Build history of the part. All positions in model axes, mm. Face numbers are marked on the shaded views. A direction names the side the tool comes from. Give positions to 0.01 mm unless a question says otherwise; leave off trailing zeros. Order: outer loops, then holes, each group sorted by start corner. A loop starts at its lowest first (then second) coordinate and runs counter-clockwise, first axis right, second up. Notation, with made-up numbers: (2.5, 76.5) - (47.5, 76.5) arc R10 ccw to (47.5, 83.5) - close; hole circle Ø2 at (13, 10.25). An arc over 180 degrees is marked (long way). Write each question's results on one line, items separated by ' | '. Start each with the question number.
1) Drill centre lines: line 1 along Z through (x, y) = (19.5, 6); line 2 along Y through (x, z) = (0, 5); line 3 along X through (y, z) = (8.5, 3.5). Where is each one in solid material? Low to high. Write a range as from..to.
2) Tool access for the marked faces 1 and 2: list every direction of +Z, -Z, +X, -X, +Y, -Y with a clear straight run to the whole face (end or side of a thin tool).
3) Cut at A-A on x = 0. List the corners of the cut face in (y, z).
4) Cut at C-C on z = 23.5. List the corners of the cut face in (x, y), plus the area to 3 significant figures.
5) Drop flat-ended pins along their axis: pin 1 Ø6 at (x, z) = (9, 18.5) entering from -Y; pin 2 Ø5 at (y, z) = (-13.5, 11.5) entering from -X; pin 3 Ø4 at (y, z) = (-2.5, 6) entering from -X. Give the stop position or say it passes through.
from build123d import *

# Parameters (mm, degrees)
F0_R     = 24.25
F1_DEPTH = 25
F2_R     = 14.75
F3_DEPTH = 4.5
F4_SIZE  = 1


with BuildPart() as f1:
    # F0 (on Top) → F1 (new body)
    with BuildSketch(Plane.XY):
        Circle(F0_R)
    extrude(amount=F1_DEPTH)

    # F2 (on face) → F3 (join)
    with BuildSketch(Plane.XY.offset(25)):
        Circle(F2_R)
    extrude(amount=F3_DEPTH)

    # F4
    f4_edges = [f1.edges().sort_by_distance(p)[0] for p in [
        (-14.75, 0, 29.5),
        (-24.25, 0, 0),
    ]]
    chamfer(f4_edges, length=F4_SIZE)


solid = f1.part
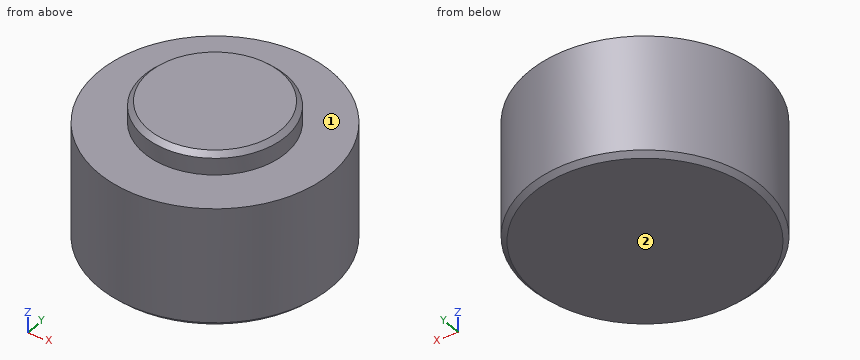
Results:
1) line 1: 0..25 | line 2: -24.25..24.25 | line 3: -22.71..22.71
2) face 1: +Z | face 2: -Z, +X, -X, +Y, -Y
3) outline: (-24.25, 1) - (-23.25, 0) - (23.25, 0) - (24.25, 1) - (24.25, 25) - (14.75, 25) - (14.75, 28.5) - (13.75, 29.5) - (-13.75, 29.5) - (-14.75, 28.5) - (-14.75, 25) - (-24.25, 25) - close
4) outline: circle Ø48.5 at (0, 0) | area: 1,850 mm^2
5) pin 1: y = -23.5 | pin 2: x = -21.61 | pin 3: x = -24.24
